```python
from build123d import *

# Parameters (mm, degrees)
ESQUISSE1_W             = 130
ESQUISSE1_H             = 100
BOSS_EXTRU_1_DEPTH      = 34
ESQUISSE2_W             = 116
ESQUISSE2_H             = 27
ENL_V_MAT_EXTRU_1_DEPTH = 106
ESQUISSE3_R             = 3.5
ENL_V_MAT_EXTRU_2_DEPTH = 10
ESQUISSE4_W             = 8
ESQUISSE4_H             = 12
ENL_V_MAT_EXTRU_3_DEPTH = 10


with BuildPart() as part:
    # Esquisse1 → Boss.-Extru.1 (new body)
    with BuildSketch(Plane.XY):
        with Locations((-0.177352831, 10.760428886)):
            Rectangle(ESQUISSE1_W, ESQUISSE1_H)
    extrude(amount=BOSS_EXTRU_1_DEPTH)

    # Esquisse2 → Enlèv. mat.-Extru.1 (cut)
    with BuildSketch(Plane.XZ.offset(39.239571114)):
        with Locations((-0.177352831, 17)):
            Rectangle(ESQUISSE2_W, ESQUISSE2_H)
    extrude(amount=-ENL_V_MAT_EXTRU_1_DEPTH, mode=Mode.SUBTRACT)

    # Esquisse3 → Enlèv. mat.-Extru.2 (cut)
    with BuildSketch(Plane.XY.offset(34)):
        with Locations((-52.677352831, 35.760428886)):
            Circle(ESQUISSE3_R)
    extrude(amount=-ENL_V_MAT_EXTRU_2_DEPTH, mode=Mode.SUBTRACT)

    # Esquisse4 → Enlèv. mat.-Extru.3 (cut)
    with BuildSketch(Plane(origin=(64.822647169, 0, 0), x_dir=(0, 0, -1), z_dir=(1, 0, 0))):
        with Locations((-25, -5.239571114)):
            Rectangle(ESQUISSE4_W, ESQUISSE4_H)
    extrude(amount=-ENL_V_MAT_EXTRU_3_DEPTH, mode=Mode.SUBTRACT)


solid = part.part
```
Model file for the job. Use its own axes, mm. A direction names the side the tool comes from. Coordinates: 2 decimals unless noted, no trailing zeros. Write each loop counter-clockwise with the first axis right and the second up, starting at its lowest first coordinate (ties: lowest second). Pieces come first, ordered by that corner, then holes. Notation, with made-up numbers: (-24, 24.5) - (-12, 24.5) arc R35 cw to (-12, 56.5) - close; hole circle Ø10 at (-26, 15). An arc over 180 degrees is marked (long way). One line per item, written item: value. Start each with the question number.
1. Tool access for faces 5 (the flat face through (61, 0.76, 25)), 6 (the flat face through (-1, 10, 3.5)), 7 (the cylindrical face through (-55.455, 33.631, 32.275)): list every direction of +Z, -Z, +X, -X, +Y, -Y with a clear straight run to the whole face (end or side of a thin tool).
2. Mould opens along X. For faces 1 (the flat face through (-10, 60.76, 31)), 2 (the flat face through (-58.177, 10, 17)), 3 (the flat face through (57.823, 10, 17)), 4 (the flat face through (-65.177, 10, 17)) say: released by +X, released by -X, zero draft, split by the parting line, or undercut.
3. Slice it at A-A (z = 27). Write the cut outline in (x, y), plus the area to 3 significant figures.
4. Flat gauge pins, fed straight in: pin 1 (5 mm diameter, centred on x = -24.5, y = 26.5, fed in from -Z); pin 2 (1.5 mm diameter, centred on x = -34, z = 29, fed in from -Y). Where does each tip first touch, or does it go through?
5. Probe line 1 (Z direction, x = 35, y = -32); line 2 (X direction, y = 34.5, z = 27). List the from-to ranges inside material, lowest first. Write a range as from..to.
6. Slice it at B-B (x = 13.5). Write the cut outline in (y, z).
7. Slice it at C-C (z = 15.5). Write the cut outline in (x, y).
8. Slice it at D-D (y = -23.5). Write the cut outline in (x, z).
Answers below:
1. face 5: +X
1. face 6: +Y, -Y
1. face 7: +Z
2. face 1: zero draft
2. face 2: undercut
2. face 3: undercut
2. face 4: released by -X
3. outline: (-65.18, -39.24) - (-58.18, -39.24) - (-58.18, 60.76) - (-65.18, 60.76) - close; (57.82, -39.24) - (64.82, -39.24) - (64.82, -11.24) - (57.82, -11.24) - close; (57.82, 0.76) - (64.82, 0.76) - (64.82, 60.76) - (57.82, 60.76) - close
3. area: 1,320 mm^2
4. pin 1: stops at z = 0
4. pin 2: passes through
5. line 1: z = 0..3.5, 30.5..34
5. line 2: x = -65.18..-58.18, 57.82..64.82
6. outline: (-39.24, 0) - (60.76, 0) - (60.76, 3.5) - (-39.24, 3.5) - close; (-39.24, 30.5) - (60.76, 30.5) - (60.76, 34) - (-39.24, 34) - close
7. outline: (-65.18, -39.24) - (-58.18, -39.24) - (-58.18, 60.76) - (-65.18, 60.76) - close; (57.82, -39.24) - (64.82, -39.24) - (64.82, 60.76) - (57.82, 60.76) - close
8. outline: (-65.18, 0) - (64.82, 0) - (64.82, 34) - (-65.18, 34) - close; hole (-58.18, 3.5) - (57.82, 3.5) - (57.82, 30.5) - (-58.18, 30.5) - close
